Could you check a few things on this model? Use its own coordinates, in mm. Face numbers are marked on the shaded views. A direction names the side the tool comes from. Round coordinates to 2 decimals unless told otherwise and drop trailing zeros. Loops run counter-clockwise (first coordinate to the right, second up) from the corner with the lowest first, then second, coordinate; pieces in that order, holes last. Notation, with made-up numbers: M -35.75,55.25 L 15.25,55.25 A16 ccw 15.25,59.25 Z; hole C 54.5,1 d8. An arc over 180 degrees is marked long. Answer in a Markdown table with one row per item.
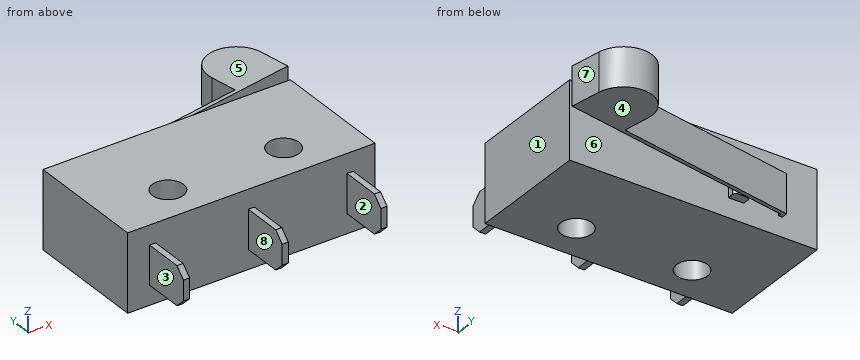
```python
from build123d import *

# Parameters (mm, degrees)
SKETCH1_W           = 20.32
SKETCH1_H           = 6.35
BOSS_EXTRUDE1_DEPTH = 10
SKETCH2_W           = 0.5
SKETCH2_H           = 4
BOSS_EXTRUDE2_DEPTH = 1.5875
CHAMFER1_SIZE       = 0.762
SKETCH3_R           = 1.275
CUT_EXTRUDE1_DEPTH  = 23.934585372


with BuildPart() as part:
    # Sketch1 → Boss-Extrude1 (new body)
    with BuildSketch(Plane(origin=(0, 0, 0), x_dir=(1, 0, 0), z_dir=(0, 1, 0))):
        Rectangle(SKETCH1_W, SKETCH1_H)
    extrude(amount=BOSS_EXTRUDE1_DEPTH)

    # Sketch2 → Boss-Extrude2 (add, symmetric)
    with BuildSketch(Plane.XY):
        with BuildLine():
            Line((-4.1425, 10), (-4.1425, 10.508))
            ThreePointArc((-4.1425, 10.508), (-4.068105122, 10.687605122), (-3.8885, 10.762))
            Line((-3.8885, 10.762), (-3.1265, 10.762))
            ThreePointArc((-3.1265, 10.762), (-2.946894878, 10.687605122), (-2.8725, 10.508))
            Line((-2.8725, 10.508), (-2.8725, 10))
            Line((-2.8725, 10), (-4.1425, 10))
        make_face()
        with BuildLine():
            Line((-7.31, 10), (-7.31, 10.520414133))
            Line((-7.31, 10.520414133), (7.835766275, 13.191021371))
            Line((7.835766275, 13.191021371), (7.4498332, 15.379756602))
            ThreePointArc((7.4498332, 15.379756602), (9.355652622, 18.101548811), (12.077444831, 16.195729389))
            Line((12.077444831, 16.195729389), (12.518511203, 13.694317696))
            Line((12.518511203, 13.694317696), (-6.9925, 10.254))
            Line((-6.9925, 10.254), (-6.9925, 10))
            Line((-6.9925, 10), (-7.31, 10))
        make_face()
        with Locations((-8.11, -2)):
            Rectangle(SKETCH2_W, SKETCH2_H)
        with Locations((0, -2)):
            Rectangle(SKETCH2_W, SKETCH2_H)
        with Locations((8.11, -2)):
            Rectangle(SKETCH2_W, SKETCH2_H)
    extrude(amount=BOSS_EXTRUDE2_DEPTH, both=True)

    # Chamfer1
    chamfer1_edges = [part.edges().sort_by_distance(p)[0] for p in [
        (-8.11, -4, -1.5875),
        (-8.11, -4, 1.5875),
        (0, -4, -1.5875),
        (0, -4, 1.5875),
        (8.11, -4, -1.5875),
        (8.11, -4, 1.5875),
    ]]
    chamfer(chamfer1_edges, length=CHAMFER1_SIZE)

    # Sketch3 → Cut-Extrude1 (cut, through all)
    with BuildSketch(Plane.XY.offset(3.175)):
        with Locations((-4.75, 3.025)):
            Circle(SKETCH3_R)
        with Locations((4.75, 3.025)):
            Circle(SKETCH3_R)
    extrude(amount=-CUT_EXTRUDE1_DEPTH, mode=Mode.SUBTRACT)


solid = part.part
```
1) I need wall thicknesses on line 1 (X direction, y = -1.5, z = 0); line 2 (Y direction, x = 4.75, z = 0); line 3 (Y direction, x = -5.25, z = 1.5). Which ranges of each line are inside material? Lowest first, please.
Computed:
| item | result |
|---|---|
| line 1 | x = -8.36 to -7.86, -0.25 to 0.25, 7.86 to 8.36 |
| line 2 | y = 0 to 1.75, 4.3 to 10, 12.32 to 12.65 |
| line 3 | y = 0 to 1.85, 4.2 to 10, 10.56 to 10.88 |
2) If we mould it in two halves opening along Y, with no side actions, what happens to the marked faces 6, 7 and 8? For each: released by +Y, released by -Y, zero draft, split by the parting line, or undercut.
Computed:
| item | result |
|---|---|
| face 6 | undercut |
| face 7 | released by +Y |
| face 8 | zero draft |
3) I want a section at B-B, the plane x = -4.75. State how many separate pieces and enclosed holes the cut face has, plus the area to 3 significant figures.
Computed:
| item | result |
|---|---|
| separate pieces | 3 |
| enclosed holes | 0 |
| area | 48.3 mm² |
4) I want a section at D-D, the plane y = 1.25. Please give me the cut outline in (x, z) (3 decimals).
Computed:
| item | result |
|---|---|
| outline | M -10.16,-3.175 L 10.16,-3.175 L 10.16,3.175 L -10.16,3.175 Z |
5) Which directions (+Z, -Z, +X, -X, +Y, -Y) give clear straight access to the entire face, cutting with the end or side of a thin tool? Please do the marked faces 1, 2, 3, 4 and 5.
Computed:
| item | result |
|---|---|
| face 1 | +Z, -Z, +X, -Y |
| face 2 | +Z, -Z, -Y |
| face 3 | +Z, -Z, -X, -Y |
| face 4 | -Z, +X, -X, +Y |
| face 5 | +Z, +X, -X, +Y |
6) I want a section at C-C, the plane z = 2. Please give me the cut outline in (x, y) (3 decimals).
Computed:
| item | result |
|---|---|
| outline | M -10.16,0 L 10.16,0 L 10.16,10 L -10.16,10 Z; hole C -4.75,3.025 d2.55; hole C 4.75,3.025 d2.55 |
7) I want a section at A-A, the plane y = -2. Please give me the cut outline in (x, z), plus the area to 3 significant figures.
Computed:
| item | result |
|---|---|
| outline | M -8.36,-1.59 L -7.86,-1.59 L -7.86,1.59 L -8.36,1.59 Z; M -0.25,-1.59 L 0.25,-1.59 L 0.25,1.59 L -0.25,1.59 Z; M 7.86,-1.59 L 8.36,-1.59 L 8.36,1.59 L 7.86,1.59 Z |
| area | 4.76 mm² |
8) Will these pins go through, and if not, where does the flat tip stop? P1, Ø2.5, axis at y = -2.5, z = 1, coming from the +X side; P2, Ø0.8, axis at x = -3.5, y = 10.5, coming from the -Z side; P3, Ø0.6, axis at x = -8, y = -1.5, coming from the +Z side; P4, Ø2, axis at x = -4.75, y = 3.025, coming from the +Z side.
Computed:
| item | result |
|---|---|
| P1 | stops at x = 8.36 |
| P2 | stops at z = -1.59 |
| P3 | stops at z = 1.59 |
| P4 | passes through |
